Autodesk Inventor part; units mm, degrees
ref_plane "YZ Plane" through (0, 0, 0) normal (1, 0, 0) x (0, 1, 0)
ref_plane "XZ Plane" through (0, 0, 0) normal (0, 1, 0) x (-1, 0, 0)
ref_plane "XY Plane" through (0, 0, 0) normal (0, 0, 1) x (1, 0, 0)
sketch "Sketch1" plane through (0, 0, 0) normal (1, 0, 0) x (0, 1, 0)
  line L0 (-10.311, 3.6207) -> (-11.2914, 1.5298)
  line L1 (-11.2914, 1.5298) -> (-13.5924, 1.3333)
  line L2 (-13.5924, 1.3333) -> (-14.913, 3.2279)
  line L3 (-14.913, 3.2279) -> (-13.9326, 5.3188)
  line L4 (-13.9326, 5.3188) -> (-11.6316, 5.5153)
  line L5 (-11.6316, 5.5153) -> (-10.311, 3.6207)
  point P0 (0, 0)
  point P1 (-12.612, 3.4243)
  dimension "d0" = 2
extrude "Extrusion1" add sketch "Sketch1" along normal blind 8
sketch "Sketch2" plane through (8, 0, 0) normal (1, 0, 0) x (0, 0, -1)
  line L0 (-3.6207, -10.311) -> (-5.5153, -11.6316)
  line L1 (-3.2279, -14.913) -> (-1.3333, -13.5924)
  line L2 (-4.568, -10.9713) -> (-2.2806, -14.2527)
  circle A0 centre (-3.4243, -12.612) radius 1.25
  point P0 (0, 0)
  dimension "d3" = 2.5
extrude "Extrusion2" add sketch "Sketch2" along normal blind 6
thread "Thread1"
sketch "Sketch3" plane through (0, 0, 0) normal (-1, 0, 0) x (0, 0, 1)
  line L0 (1.3333, -13.5924) -> (3.2279, -14.913)
  line L1 (5.5153, -11.6316) -> (3.6207, -10.311)
  line L2 (4.568, -10.9713) -> (2.2806, -14.2527)
  point P0 (0, 0)
  point P1 (3.4243, -12.612)
hole "Hole1" at (0, -12.612, 3.4243) direction (1, 0, 0) diameter 2.013 depth 5 tip angle 118
properties part number "standoff" material "Brass, Soft Yellow"
Verification items for the finished model (mm, model axes). A direction names the side the tool comes from. Give positions to 0.01 mm unless a question says otherwise; leave off trailing zeros. Order: outer loops, then holes, each group sorted by start corner. A loop starts at its lowest first (then second) coordinate and runs counter-clockwise, first axis right, second up. Notation, with made-up numbers: (-38, -20.75) -> (3, -20.75) arc R16 ccw to (3, -1.75) -> close; hole circle Ø11 at (-0.5, 57). An arc over 180 degrees is marked (long way). Use a Markdown table: item, result.
1) Tool access check on faces 4 (the flat face through (3.944, -12.798, 5.416)), 5 (the cylindrical face through (10.958, -13.457, 4.346)). Record the directions out of +Z, -Z, +X, -X, +Y, -Y that give a thin tool (end or side, any length) a straight path to the whole face; none if there is none.
Results:
| item | result |
|---|---|
| face 4 | +Z, +X, -X, -Y |
| face 5 | +X |
2) Material ranges on probe 1 along X at (y, z) = (-11.6, 4.35); probe 2 along Y at (x, z) = (12, 3.45); probe 3 along Z at (x, y) = (10, -12.55), recorded low to high.
Results:
| item | result |
|---|---|
| probe 1 | 0 to 8 |
| probe 2 | -13.86 to -11.36 |
| probe 3 | 2.18 to 4.67 |
3) Section check B-B, the plane x = 7. Record the boundary of the cut face in (y, z), then the cut area to 3 significant figures.
Results:
| item | result |
|---|---|
| outline | (-14.91, 3.23) -> (-13.59, 1.33) -> (-11.29, 1.53) -> (-10.31, 3.62) -> (-11.63, 5.52) -> (-13.93, 5.32) -> close |
| area | 13.9 mm² |
4) Section check A-A, the plane x = 2.5. Record the boundary of the cut face in (y, z).
Results:
| item | result |
|---|---|
| outline | (-14.91, 3.23) -> (-13.59, 1.33) -> (-11.29, 1.53) -> (-10.31, 3.62) -> (-11.63, 5.52) -> (-13.93, 5.32) -> close; hole circle Ø2.01 at (-12.61, 3.42) |
5) Section check D-D, the plane z = 2. Record the boundary of the cut face in (x, y).
Results:
| item | result |
|---|---|
| outline | (0, -14.06) -> (8, -14.06) -> (8, -11.07) -> (0, -11.07) -> close |
6) Depth check by flat-ended pin: pin 1 Ø1.5 at (x, y) = (7, -13.5) entering from +Z; pin 2 Ø1 at (x, y) = (7.5, -12) entering from -Z. Enter the tip coordinate at first touch or a pass-through.
Results:
| item | result |
|---|---|
| pin 1 | z = 5.42 |
| pin 2 | z = 1.43 |
7) Mould release check, pull along Z, two halves, no side actions. Record for faces 1 (the flat face through (3.944, -10.794, 2.59)), 2 (the flat face through (0, -14, 3)), 3 (the cylindrical face through (2.54, -11.63, 3.21)): pulls with the +Z half, pulls with the -Z half, needs draft (parallel to the pull), parting line crosses it, or undercut.
Results:
| item | result |
|---|---|
| face 1 | pulls with the -Z half |
| face 2 | needs draft |
| face 3 | undercut |
8) Section check C-C, the plane y = -14.4. Record the boundary of the cut face in (x, z), then the cut area to 3 significant figures.
Results:
| item | result |
|---|---|
| outline | (0, 2.49) -> (8, 2.49) -> (8, 4.32) -> (0, 4.32) -> close |
| area | 14.6 mm² |
